Verification items for the finished model (mm, model axes). Coordinates: 2 decimals unless noted, no trailing zeros. Loops run counter-clockwise (first coordinate to the right, second up) from the corner with the lowest first, then second, coordinate; pieces in that order, holes last. Notation, with made-up numbers: (17, 70.25) -> (34, 70.25) arc R10 ccw to (34, 87.25) -> close; hole circle Ø2 at (73, -9.5). An arc over 180 degrees is marked (long way). Answer as a JSON object with one key per item and string values. Group by question number.
Q1. Cross-section at C-C on y = 1. Record the boundary of the cut face in (x, z), and give its area (3 significant figures).
Q2. Gauge pin test, flat end, axial feed: pin 1 Ø5 at (x, y) = (-1, 12.5) entering from -Z. Record the tip position at first contact, or that the pin passes through.
Q3. Cross-section at A-A on x = 0. Record the boundary of the cut face in (y, z).
Q4. Cross-section at D-D on x = 3. Record the boundary of the cut face in (y, z), and give its area (3 significant figures).
Q5. Release check for a two-part mould opening along X. For faces 1 (the flat face through (5.5, 7, 1)), 2 (the cylindrical face through (-0.29, 2.23, 1.48)), 3 (the flat face through (-5.5, 7, 1)) record: released by +X, released by -X, zero draft, split by the parting line, or undercut.
Q6. Cross-section at B-B on z = 1.15. Record the boundary of the cut face in (x, y).
Q7. Scan lines: L1, parallel to Y at x = 0, z = 0.6; L2, parallel to X at y = -1.75, z = 1.4; L3, parallel to Y at x = 0.75, z = 0.85. Record each from-to range of solid material in increasing order.
```python
from build123d import *

# Parameters (mm, degrees)
F0_R     = 2.25
F1_DEPTH = 3


with BuildPart() as f1:
    # F0 (on Top) → F1 (new body)
    with BuildSketch(Plane.XY):
        with BuildLine():
            Line((-5.5, 14), (-5.5, 0))
            ThreePointArc((-5.5, 0), (0, -5.5), (5.5, 0))
            Line((5.5, 0), (5.5, 14))
            ThreePointArc((5.5, 14), (5.207107, 14.707107), (4.5, 15))
            Line((4.5, 15), (-4.5, 15))
            ThreePointArc((-4.5, 15), (-5.207107, 14.707107), (-5.5, 14))
        make_face()
        Circle(F0_R, mode=Mode.SUBTRACT)
    extrude(amount=F1_DEPTH)


solid = f1.part
```
Computed values:
{
 "1": {"outline": "(-5.5, 0) -> (-2.02, 0) -> (-2.02, 3) -> (-5.5, 3) -> close; (2.02, 0) -> (5.5, 0) -> (5.5, 3) -> (2.02, 3) -> close", "area": "20.9 mm²"},
 "2": {"pin 1": "stops at z = 0"},
 "3": {"outline": "(-5.5, 0) -> (-2.25, 0) -> (-2.25, 3) -> (-5.5, 3) -> close; (2.25, 0) -> (15, 0) -> (15, 3) -> (2.25, 3) -> close"},
 "4": {"outline": "(-4.61, 0) -> (15, 0) -> (15, 3) -> (-4.61, 3) -> close", "area": "58.8 mm²"},
 "5": {"face 1": "released by +X", "face 2": "undercut", "face 3": "released by -X"},
 "6": {"outline": "(-5.5, 0) arc R5.5 ccw to (5.5, 0) -> (5.5, 14) arc R1 ccw to (4.5, 15) -> (-4.5, 15) arc R1 ccw to (-5.5, 14) -> close; hole circle Ø4.5 at (0, 0)"},
 "7": {"L1": "y = -5.5 to -2.25, 2.25 to 15", "L2": "x = -5.21 to -1.41, 1.41 to 5.21", "L3": "y = -5.45 to -2.12, 2.12 to 15"}
}
